The listing builds one solid part. Answer for the finished solid, in the listing's coordinates (mm). Face numbers are marked on the shaded views. Give positions to 0.01 mm unless a question says otherwise; leave off trailing zeros. Loops run counter-clockwise (first coordinate to the right, second up) from the corner with the lowest first, then second, coordinate; pieces in that order, holes last.
Item 1: Section D-D, the plane x = -63 is taken. Give the vertices of the cut face in (y, z), and give its area (3 significant figures).
Item 2: Section A-A, the plane x = 16 is taken. Give the vertices of the cut face in (y, z).
Item 3: Consider line 1 along X through (y, z) = (84.5, 1); line 2 along Y through (x, z) = (6, 1.5); line 3 along X through (y, z) = (108, 10.5). Determine where each line is inside the solid, lowest interval first.
Item 4: Each of these flat-tipped pins is pushed along its axis until it touches: pin 1 Ø11 at (x, z) = (-73.5, 17) entering from +Y; pin 2 Ø1 at (y, z) = (15, 21) entering from +X; pin 3 Ø1.5 at (x, z) = (-58, 3) entering from +Y; pin 4 Ø3 at (x, y) = (86.5, 33) entering from +Z. Where does it stop, or does it pass through?
Item 5: Section B-B, the plane y = 107 is taken. Give the vertices of the cut face in (x, z), and give its area (3 significant figures).
Item 6: Section C-C, the plane y = 200.5 is taken. Give the vertices of the cut face in (x, z).
Item 7: The mould has two halves that part along X. Classify the marked faces 1, 2 and 3: pulls with the +X half, pulls with the -X half, needs draft (parallel to the pull), parting line crosses it, or undercut.
from build123d import *
from OCP.BRepFilletAPI import BRepFilletAPI_MakeChamfer

# Parameters (mm, degrees)
BOSS_EXTRUDE1_DEPTH             = 10
BOSS_EXTRUDE2_DEPTH             = 10
SKETCH3_W                       = 9
SKETCH3_H                       = 9
BOSS_EXTRUDE3_DEPTH             = 10
SKETCH5_W                       = 9
SKETCH5_H                       = 9
BOSS_EXTRUDE4_DEPTH             = 10
SKETCH6_R                       = 2.25
CUT_EXTRUDE1_DEPTH              = 9
SKETCH7_R                       = 2.25
CUT_EXTRUDE2_DEPTH              = 9
SKETCH8_R                       = 1.75
CUT_EXTRUDE3_DEPTH              = 250.05692246
CUT_EXTRUDE4_DEPTH              = 2.1
SKETCH10_W                      = 9
SKETCH10_H                      = 9
CUT_EXTRUDE5_DEPTH              = 12
SKETCH11_R                      = 1.8
CUT_EXTRUDE6_DEPTH              = 10
CHAMFER1_SIZE                   = 0.5
CHAMFER1_SIZE2                  = 1.866025404
CUT_EXTRUDE7_DEPTH              = 2.1
CUT_EXTRUDE8_DEPTH              = 2.1
SKETCH14_W                      = 120
SKETCH14_H                      = 20
BOSS_EXTRUDE5_DEPTH             = 5.84
BOSS_EXTRUDE5_DIRECTION_2_REACH = 232.648
CUT_EXTRUDE9_START              = -20
SKETCH15_W                      = 80
SKETCH15_H                      = 7
CUT_EXTRUDE9_DEPTH              = 20
CUT_EXTRUDE10_START             = -15.84
CUT_EXTRUDE10_DEPTH             = 22.84
SKETCH17_W                      = 8
SKETCH17_H                      = 15.5
BOSS_EXTRUDE6_DEPTH             = 2


with BuildPart() as part:
    # Sketch1 → Boss-Extrude1 (new body)
    with BuildSketch(Plane.XY):
        Polygon((0, 0), (-91.5, 0), (-91.5, 220.775), (-71.5, 220.775), (-71.5, 40), (-51.5, 20), (0, 20), (51.5, 20), (71.5, 40), (71.5, 140.775), (91.5, 140.775), (91.5, 0), align=None)
    extrude(amount=BOSS_EXTRUDE1_DEPTH)

    # Sketch2 → Boss-Extrude2 (add)
    with BuildSketch(Plane.XY.offset(10)):
        Polygon((-81.5, 220.775), (-91.5, 220.775), (-91.5, 0), (91.5, 0), (91.5, 140.775), (81.5, 140.775), (81.5, 10), (-81.5, 10), align=None)
    extrude(amount=BOSS_EXTRUDE2_DEPTH)

    # Sketch3 → Boss-Extrude3 (add)
    with BuildSketch(Plane(origin=(0, 220.775, 0), x_dir=(1, 0, 0), z_dir=(0, 1, 0))):
        with Locations((-87, -4.5)):
            Rectangle(SKETCH3_W, SKETCH3_H)
    extrude(amount=BOSS_EXTRUDE3_DEPTH)

    # Sketch5 → Boss-Extrude4 (add)
    with BuildSketch(Plane(origin=(0, 140.775, 0), x_dir=(1, 0, 0), z_dir=(0, 1, 0))):
        with Locations((87, -4.5)):
            Rectangle(SKETCH5_W, SKETCH5_H)
    extrude(amount=BOSS_EXTRUDE4_DEPTH)

    # Sketch6 → Cut-Extrude1 (cut)
    with BuildSketch(Plane.ZY.offset(91.5)):
        with Locations(Location((4.5, 225.775, 0), (0, 0, 270))):
            Circle(SKETCH6_R)
    extrude(amount=-CUT_EXTRUDE1_DEPTH, mode=Mode.SUBTRACT)

    # Sketch7 → Cut-Extrude2 (cut)
    with BuildSketch(Plane(origin=(91.5, 0, 0), x_dir=(0, 0, -1), z_dir=(1, 0, 0))):
        with Locations(Location((-4.5, 145.775, 0), (0, 0, 90))):
            Circle(SKETCH7_R)
    extrude(amount=-CUT_EXTRUDE2_DEPTH, mode=Mode.SUBTRACT)

    # Sketch8 → Cut-Extrude3 (cut, through all)
    with BuildSketch(Plane(origin=(0, 0, 0), x_dir=(-1, 0, 0), z_dir=(0, 0, -1))):
        with Locations((86.5, 33)):
            Circle(SKETCH8_R)
        with Locations((-86.5, 33)):
            Circle(SKETCH8_R)
    extrude(amount=-CUT_EXTRUDE3_DEPTH, mode=Mode.SUBTRACT)

    # Sketch9 → Cut-Extrude4 (cut)
    with BuildSketch(Plane(origin=(0, 0, 0), x_dir=(-1, 0, 0), z_dir=(0, 0, -1))):
        Polygon((-84.854551733, 30.15), (-83.209103466, 33), (-84.854551733, 35.85), (-88.145448267, 35.85), (-89.790896534, 33), (-88.145448267, 30.15), align=None)
        Polygon((88.145448267, 30.15), (89.790896534, 33), (88.145448267, 35.85), (84.854551733, 35.85), (83.209103466, 33), (84.854551733, 30.15), align=None)
    extrude(amount=-CUT_EXTRUDE4_DEPTH, mode=Mode.SUBTRACT)

    # Sketch10 → Cut-Extrude5 (cut)
    with BuildSketch(Plane.XY.offset(20)):
        with Locations((87, 4.5)):
            Rectangle(SKETCH10_W, SKETCH10_H)
        with Locations((-87, 4.5)):
            Rectangle(SKETCH10_W, SKETCH10_H)
    extrude(amount=-CUT_EXTRUDE5_DEPTH, mode=Mode.SUBTRACT)

    # Sketch11 → Cut-Extrude6 (cut)
    with BuildSketch(Plane.XZ.offset(-9)):
        with Locations(Location((-87, 14, 0), (0, 0, 270))):
            Circle(SKETCH11_R)
        with Locations(Location((87, 14, 0), (0, 0, 270))):
            Circle(SKETCH11_R)
    extrude(amount=-CUT_EXTRUDE6_DEPTH, mode=Mode.SUBTRACT)

    # Chamfer1: one chamfer whose edges measure the first distance from different faces: ONE call of the kernel's chamfer builder (chamfer() names one face for all edges)
    chamfer1_edges_1 = [part.edges().sort_by_distance(p)[0] for p in [
        (-87, 9, 15.8),
    ]]
    chamfer1_side_1 = [part.faces().sort_by_distance(p)[0] for p in [
        (-91.35, 9, 14),
    ]]
    chamfer1_edges_2 = [part.edges().sort_by_distance(p)[0] for p in [
        (87, 9, 15.8),
    ]]
    chamfer1_side_2 = [part.faces().sort_by_distance(p)[0] for p in [
        (82.65, 9, 14),
    ]]
    chamfer1 = BRepFilletAPI_MakeChamfer(part.part.solid().wrapped)
    for e in chamfer1_edges_1:
        chamfer1.Add(CHAMFER1_SIZE, CHAMFER1_SIZE2, e.wrapped, chamfer1_side_1[0].wrapped)  # the first distance lies on this face
    for e in chamfer1_edges_2:
        chamfer1.Add(CHAMFER1_SIZE, CHAMFER1_SIZE2, e.wrapped, chamfer1_side_2[0].wrapped)  # the first distance lies on this face
    add(Compound.cast(chamfer1.Shape()), mode=Mode.REPLACE)

    # Sketch12 → Cut-Extrude7 (cut)
    with BuildSketch(Plane.ZY.offset(91.5)):
        Polygon((6.145448267, 222.925), (7.790896534, 225.775), (6.145448267, 228.625), (2.854551733, 228.625), (1.209103466, 225.775), (2.854551733, 222.925), align=None)
    extrude(amount=-CUT_EXTRUDE7_DEPTH, mode=Mode.SUBTRACT)

    # Sketch13 → Cut-Extrude8 (cut)
    with BuildSketch(Plane(origin=(91.5, 0, 0), x_dir=(0, 0, -1), z_dir=(1, 0, 0))):
        Polygon((-2.854551733, 142.925), (-1.209103466, 145.775), (-2.854551733, 148.625), (-6.145448267, 148.625), (-7.790896534, 145.775), (-6.145448267, 142.925), align=None)
    extrude(amount=-CUT_EXTRUDE8_DEPTH, mode=Mode.SUBTRACT)

    # Sketch14 → Boss-Extrude5 (add)
    with BuildSketch(Plane(origin=(0, 20, 0), x_dir=(1, 0, 0), z_dir=(0, 1, 0))):
        with Locations((0, -10)):
            Rectangle(SKETCH14_W, SKETCH14_H)
        with BuildLine():
            Line((-50, -7.65), (20, -7.65))
            ThreePointArc((20, -7.65), (22.35, -10), (20, -12.35))
            Line((20, -12.35), (-50, -12.35))
            ThreePointArc((-50, -12.35), (-52.35, -10), (-50, -7.65))
        make_face(mode=Mode.SUBTRACT)
    extrude(amount=BOSS_EXTRUDE5_DEPTH)

    # Boss-Extrude5 direction 2: up to this face of the body (flat: up to its plane)
    boss_extrude5_direction_2_end = Plane(part.part.faces().sort_by_distance((0, 10, 15))[0])
    # Sketch14 → Boss-Extrude5 direction 2 (add, up to the picked face)
    with BuildSketch(Plane(origin=(0, 20, 0), x_dir=(1, 0, 0), z_dir=(0, 1, 0)), mode=Mode.PRIVATE) as boss_extrude5_direction_2_sk1:
        with Locations((0, -10)):
            Rectangle(SKETCH14_W, SKETCH14_H)
        with BuildLine():
            Line((-50, -7.65), (20, -7.65))
            ThreePointArc((20, -7.65), (22.35, -10), (20, -12.35))
            Line((20, -12.35), (-50, -12.35))
            ThreePointArc((-50, -12.35), (-52.35, -10), (-50, -7.65))
        make_face(mode=Mode.SUBTRACT)
    boss_extrude5_direction_2_tool1 = split(extrude(boss_extrude5_direction_2_sk1.sketch, amount=-BOSS_EXTRUDE5_DIRECTION_2_REACH, mode=Mode.PRIVATE), bisect_by=boss_extrude5_direction_2_end, keep=Keep.BOTH, mode=Mode.PRIVATE)
    add(boss_extrude5_direction_2_tool1.solids().sort_by(Axis((0, 20, 18.783447), (0, -1, 0)))[0])

    # Sketch15 → Cut-Extrude9 (cut)
    with BuildSketch(Plane(origin=(0, 0, 0), x_dir=(-1, 0, 0), z_dir=(0, 0, -1)).offset(CUT_EXTRUDE9_START)):
        with Locations((10, 19.34)):
            Rectangle(SKETCH15_W, SKETCH15_H)
    extrude(amount=CUT_EXTRUDE9_DEPTH, mode=Mode.SUBTRACT)

    # Sketch16 → Cut-Extrude10 (cut)
    with BuildSketch(Plane(origin=(0, 15.84, 0), x_dir=(1, 0, 0), z_dir=(0, 1, 0)).offset(CUT_EXTRUDE10_START)):
        with BuildLine():
            Line((20, -5.3), (-50, -5.3))
            ThreePointArc((-50, -5.3), (-54.7, -10), (-50, -14.7))
            Line((-50, -14.7), (20, -14.7))
            ThreePointArc((20, -14.7), (24.7, -10), (20, -5.3))
        make_face()
    extrude(amount=CUT_EXTRUDE10_DEPTH, mode=Mode.SUBTRACT)

    # Sketch17 → Boss-Extrude6 (add)
    with BuildSketch(Plane.XY.offset(20)):
        with Locations((-25, 18.09)):
            Rectangle(SKETCH17_W, SKETCH17_H)
        with Locations((5, 18.09)):
            Rectangle(SKETCH17_W, SKETCH17_H)
    extrude(amount=BOSS_EXTRUDE6_DEPTH)


solid = part.part
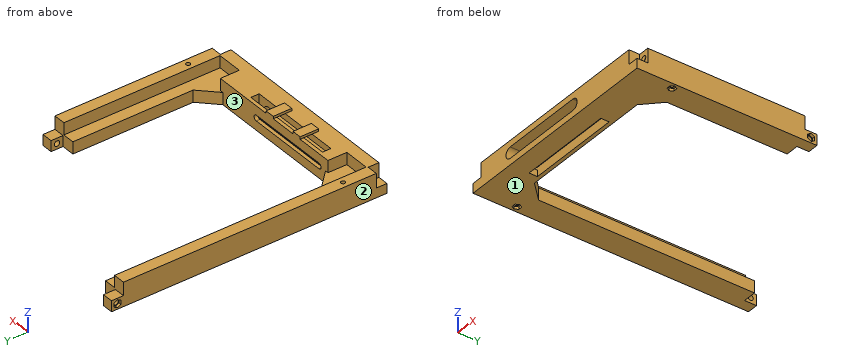
Worked answers:
1. outline: (0, 0) - (31.5, 0) - (31.5, 10) - (10, 10) - (10, 20) - (0, 20) - close
1. area: 415 mm2
2. outline: (0, 0) - (15.84, 0) - (15.84, 5.3) - (0, 5.3) - close; (0, 14.7) - (15.84, 14.7) - (15.84, 20) - (0, 20) - close; (22.84, 0) - (25.84, 0) - (25.84, 7.65) - (22.84, 7.65) - close; (22.84, 12.35) - (25.84, 12.35) - (25.84, 20) - (22.84, 20) - close
3. line 1: x = -91.5 to -71.5, 71.5 to 91.5
3. line 2: y = 0 to 15.84, 22.84 to 25.84
3. line 3: x = -91.5 to -81.5, 81.5 to 91.5
4. pin 1: stops at y = 10
4. pin 2: stops at x = 9
4. pin 3: stops at y = 27.25
4. pin 4: passes through
5. outline: (-91.5, 0) - (-71.5, 0) - (-71.5, 10) - (-81.5, 10) - (-81.5, 20) - (-91.5, 20) - close; (71.5, 0) - (91.5, 0) - (91.5, 20) - (81.5, 20) - (81.5, 10) - (71.5, 10) - close
5. area: 600 mm2
6. outline: (-91.5, 0) - (-71.5, 0) - (-71.5, 10) - (-81.5, 10) - (-81.5, 20) - (-91.5, 20) - close
7. face 1: needs draft
7. face 2: pulls with the -X half
7. face 3: undercut
